Build history of the part. All positions in model axes, mm. A direction names the side the tool comes from. Give positions to 0.01 mm unless a question says otherwise; leave off trailing zeros. Loops run counter-clockwise (first coordinate to the right, second up) from the corner with the lowest first, then second, coordinate; pieces in that order, holes last. Notation, with made-up numbers: M 24.25,4 L 72.25,4 A25 ccw 72.25,39 Z; hole C 53.25,-40 d9. An arc over 180 degrees is marked long. Answer in a Markdown table with one row per item. Add a question column.
```python
from build123d import *

# Parameters (mm, degrees)
SKETCH1_W           = 200
SKETCH1_H           = 60
BOSS_EXTRUDE1_DEPTH = 10
SKETCH2_W           = 200
SKETCH2_H           = 10
BOSS_EXTRUDE2_DEPTH = 140
SKETCH3_R           = 15.5
CUT_EXTRUDE1_DEPTH  = 60
SKETCH7_W           = 10
SKETCH7_H           = 30
CUT_EXTRUDE4_DEPTH  = 30
SKETCH9_R           = 1.5
SKETCH9_R_2         = 2.5
CUT_EXTRUDE6_DEPTH  = 20
SKETCH10_W          = 33.76561095
SKETCH10_H          = 62.627783557
CUT_EXTRUDE7_DEPTH  = 130
SKETCH11_W          = 8
SKETCH11_H          = 30
CUT_EXTRUDE8_DEPTH  = 30


with BuildPart() as part:
    # Sketch1 → Boss-Extrude1 (new body)
    with BuildSketch(Plane.XY):
        Rectangle(SKETCH1_W, SKETCH1_H)
    extrude(amount=BOSS_EXTRUDE1_DEPTH)

    # Sketch2 → Boss-Extrude2 (add)
    with BuildSketch(Plane(origin=(0, 0, 0), x_dir=(-1, 0, 0), z_dir=(0, 0, -1))):
        with Locations((0, -25)):
            Rectangle(SKETCH2_W, SKETCH2_H)
    extrude(amount=BOSS_EXTRUDE2_DEPTH)

    # Sketch3 → Cut-Extrude1 (cut)
    with BuildSketch(Plane.XY.offset(10)):
        with Locations((0, 5)):
            Circle(SKETCH3_R)
        with Locations((60, 5)):
            Circle(SKETCH3_R)
        with Locations((-60, 5)):
            Circle(SKETCH3_R)
    extrude(amount=-CUT_EXTRUDE1_DEPTH, mode=Mode.SUBTRACT)

    # Sketch7 → Cut-Extrude4 (cut)
    with BuildSketch(Plane(origin=(0, -20, 0), x_dir=(1, 0, 0), z_dir=(0, 1, 0))):
        with Locations((9, 65)):
            Rectangle(SKETCH7_W, SKETCH7_H)
        with Locations((-9, 65)):
            Rectangle(SKETCH7_W, SKETCH7_H)
    extrude(amount=-CUT_EXTRUDE4_DEPTH, mode=Mode.SUBTRACT)

    # Sketch9 → Cut-Extrude6 (cut)
    with BuildSketch(Plane(origin=(0, -20, 0), x_dir=(1, 0, 0), z_dir=(0, 1, 0))):
        with Locations(Location((-27, 80, 0), (0, 0, 270))):
            Circle(SKETCH9_R)
        with Locations(Location((27, 80, 0), (0, 0, 270))):
            Circle(SKETCH9_R)
        with Locations(Location((27, 50, 0), (0, 0, 270))):
            Circle(SKETCH9_R)
        with Locations(Location((-27, 50, 0), (0, 0, 270))):
            Circle(SKETCH9_R)
        with Locations(Location((-22, 72, 0), (0, 0, 270))):
            Circle(SKETCH9_R)
        with Locations(Location((-22, 58, 0), (0, 0, 270))):
            Circle(SKETCH9_R)
        with Locations(Location((22, 72, 0), (0, 0, 270))):
            Circle(SKETCH9_R)
        with Locations(Location((22, 58, 0), (0, 0, 270))):
            Circle(SKETCH9_R)
        with Locations(Location((95, -5, 0), (0, 0, 270))):
            Circle(SKETCH9_R_2)
        with Locations(Location((-95, -5, 0), (0, 0, 270))):
            Circle(SKETCH9_R_2)
    extrude(amount=-CUT_EXTRUDE6_DEPTH, mode=Mode.SUBTRACT)

    # Sketch10 → Cut-Extrude7 (cut, symmetric)
    with BuildSketch(Plane(origin=(0, 0, 0), x_dir=(0, 0, -1), z_dir=(1, 0, 0))):
        with Locations((-16.882805475, 11.313891779)):
            Rectangle(SKETCH10_W, SKETCH10_H)
    extrude(amount=CUT_EXTRUDE7_DEPTH, both=True, mode=Mode.SUBTRACT)

    # Sketch11 → Cut-Extrude8 (cut)
    with BuildSketch(Plane(origin=(0, -20, 0), x_dir=(1, 0, 0), z_dir=(0, 1, 0))):
        with Locations((0, 65)):
            Rectangle(SKETCH11_W, SKETCH11_H)
    extrude(amount=-CUT_EXTRUDE8_DEPTH, mode=Mode.SUBTRACT)


solid = part.part
```
(1) Pull direction X, two halves, no side cores. Call faces 1 (the flat face through (-100, -25, -64)), 2 (the flat face through (-1, -25, 10)), 3 (the flat face through (0, -25, -50)): +X half, -X half, draft (parallel to the pull), parting line (faces both ways), or undercut.
(2) Tool access for faces 4 (the flat face through (0, -25, -80)), 5 (the flat face through (1, -25, -140)): list every direction of +Z, -Z, +X, -X, +Y, -Y with a clear straight run to the whole face (end or side of a thin tool).
(3) Wall check: line 1 (X direction, y = -24.5, z = 5); line 2 (X direction, y = -24.25, z = -72); line 3 (Z direction, x = 12.5, y = -23.5). Give the ranges that are in metal, low to high.
(4) Slice it at A-A, the plane z = 5. Give the cut face in (x, y).
(5) Slice it at B-B, the plane y = -26.75. State how many separate pieces and enclosed holes the cut face has, then the cut area to 3 significant figures.
(6) Pin check, flat tip, straight feed: pin 1 (2.5 mm diameter, centred on x = -22, z = -58, fed in from -Y). Stop position of the tip, or through.
Solution:
| question | item | result |
|---|---|---|
| 1 | face 1 | -X half |
| 1 | face 2 | draft |
| 1 | face 3 | undercut |
| 2 | face 4 | +Y, -Y |
| 2 | face 5 | -Z, +X, -X, +Y, -Y |
| 3 | line 1 | -100 to -97.5, -92.5 to 92.5, 97.5 to 100 |
| 3 | line 2 | -100 to -23.5, -20.5 to -14, 14 to 20.5, 23.5 to 100 |
| 3 | line 3 | -140 to -80, -50 to 10 |
| 4 | outline | M -100,-30 L -97.5,-30 L -97.5,-20 L -100,-20 Z; M -92.5,-30 L 92.5,-30 L 92.5,-20 L -92.5,-20 Z; M 97.5,-30 L 100,-30 L 100,-20 L 97.5,-20 Z |
| 5 | separate pieces | 1 |
| 5 | enclosed holes | 11 |
| 5 | area | 29,100 mm^2 |
| 6 | pin 1 | through |
